Verification items for the finished model (mm, model axes). A direction names the side the tool comes from. Coordinates: 2 decimals unless noted, no trailing zeros. Order: outer loops, then holes, each group sorted by start corner. A loop starts at its lowest first (then second) coordinate and runs counter-clockwise, first axis right, second up. Notation, with made-up numbers: M -7.75,62.25 L 23.25,62.25 A17 ccw 23.25,88.25 Z; hole C 81.5,-22 d3. An arc over 180 degrees is marked long. Write item = value, one per line.
```python
from build123d import *
from OCP.BRepFilletAPI import BRepFilletAPI_MakeChamfer

# Parameters (mm, degrees)
SKETCH_1_W          = 200
SKETCH_1_H          = 230
EXTRUDE_1_DEPTH     = 20
CUT_EXTRUDE_1_REACH = 155.704
SKETCH_2_R          = 7
CHAMFER_1_SIZE      = 5
CHAMFER_1_SIZE2     = 3.501037691


with BuildPart() as part:
    # 草图1 → 凸台-拉伸1 (new body)
    with BuildSketch(Plane.XY):
        Rectangle(SKETCH_1_W, SKETCH_1_H)
    extrude(amount=EXTRUDE_1_DEPTH)

    # 草图2 → 切除-拉伸1 (cut, up to next)
    with BuildSketch(Plane.XY.offset(20), mode=Mode.PRIVATE) as cut_extrude_1_sk1:
        with Locations((-70, 95)):
            Circle(SKETCH_2_R)
    cut_extrude_1_tool1 = extrude(cut_extrude_1_sk1.sketch, amount=-CUT_EXTRUDE_1_REACH, mode=Mode.PRIVATE) & part.part
    # 草图2 → 切除-拉伸1 (cut, up to next)
    with BuildSketch(Plane.XY.offset(20), mode=Mode.PRIVATE) as cut_extrude_1_sk2:
        with Locations((0, 95)):
            Circle(SKETCH_2_R)
    cut_extrude_1_tool2 = extrude(cut_extrude_1_sk2.sketch, amount=-CUT_EXTRUDE_1_REACH, mode=Mode.PRIVATE) & part.part
    # 草图2 → 切除-拉伸1 (cut, up to next)
    with BuildSketch(Plane.XY.offset(20), mode=Mode.PRIVATE) as cut_extrude_1_sk3:
        with Locations((70, 95)):
            Circle(SKETCH_2_R)
    cut_extrude_1_tool3 = extrude(cut_extrude_1_sk3.sketch, amount=-CUT_EXTRUDE_1_REACH, mode=Mode.PRIVATE) & part.part
    # 草图2 → 切除-拉伸1 (cut, up to next)
    with BuildSketch(Plane.XY.offset(20), mode=Mode.PRIVATE) as cut_extrude_1_sk4:
        with Locations((-70, 35)):
            Circle(SKETCH_2_R)
    cut_extrude_1_tool4 = extrude(cut_extrude_1_sk4.sketch, amount=-CUT_EXTRUDE_1_REACH, mode=Mode.PRIVATE) & part.part
    # 草图2 → 切除-拉伸1 (cut, up to next)
    with BuildSketch(Plane.XY.offset(20), mode=Mode.PRIVATE) as cut_extrude_1_sk5:
        with Locations((70, 35)):
            Circle(SKETCH_2_R)
    cut_extrude_1_tool5 = extrude(cut_extrude_1_sk5.sketch, amount=-CUT_EXTRUDE_1_REACH, mode=Mode.PRIVATE) & part.part
    # 草图2 → 切除-拉伸1 (cut, up to next)
    with BuildSketch(Plane.XY.offset(20), mode=Mode.PRIVATE) as cut_extrude_1_sk6:
        with Locations((-70, -35)):
            Circle(SKETCH_2_R)
    cut_extrude_1_tool6 = extrude(cut_extrude_1_sk6.sketch, amount=-CUT_EXTRUDE_1_REACH, mode=Mode.PRIVATE) & part.part
    # 草图2 → 切除-拉伸1 (cut, up to next)
    with BuildSketch(Plane.XY.offset(20), mode=Mode.PRIVATE) as cut_extrude_1_sk7:
        with Locations((0, -95)):
            Circle(SKETCH_2_R)
    cut_extrude_1_tool7 = extrude(cut_extrude_1_sk7.sketch, amount=-CUT_EXTRUDE_1_REACH, mode=Mode.PRIVATE) & part.part
    # 草图2 → 切除-拉伸1 (cut, up to next)
    with BuildSketch(Plane.XY.offset(20), mode=Mode.PRIVATE) as cut_extrude_1_sk8:
        with Locations((-70, -95)):
            Circle(SKETCH_2_R)
    cut_extrude_1_tool8 = extrude(cut_extrude_1_sk8.sketch, amount=-CUT_EXTRUDE_1_REACH, mode=Mode.PRIVATE) & part.part
    # 草图2 → 切除-拉伸1 (cut, up to next)
    with BuildSketch(Plane.XY.offset(20), mode=Mode.PRIVATE) as cut_extrude_1_sk9:
        with Locations((70, -35)):
            Circle(SKETCH_2_R)
    cut_extrude_1_tool9 = extrude(cut_extrude_1_sk9.sketch, amount=-CUT_EXTRUDE_1_REACH, mode=Mode.PRIVATE) & part.part
    # 草图2 → 切除-拉伸1 (cut, up to next)
    with BuildSketch(Plane.XY.offset(20), mode=Mode.PRIVATE) as cut_extrude_1_sk10:
        with Locations((70, -95)):
            Circle(SKETCH_2_R)
    cut_extrude_1_tool10 = extrude(cut_extrude_1_sk10.sketch, amount=-CUT_EXTRUDE_1_REACH, mode=Mode.PRIVATE) & part.part
    # 草图2 → 切除-拉伸1 (cut, up to next)
    with BuildSketch(Plane.XY.offset(20), mode=Mode.PRIVATE) as cut_extrude_1_sk11:
        with BuildLine():
            Line((-41, 76), (41, 76))
            ThreePointArc((41, 76), (48.071067812, 73.071067812), (51, 66))
            Line((51, 66), (51, -66))
            ThreePointArc((51, -66), (48.071067812, -73.071067812), (41, -76))
            Line((41, -76), (-41, -76))
            ThreePointArc((-41, -76), (-48.071067812, -73.071067812), (-51, -66))
            Line((-51, -66), (-51, 66))
            ThreePointArc((-51, 66), (-48.071067812, 73.071067812), (-41, 76))
        make_face()
    cut_extrude_1_tool11 = extrude(cut_extrude_1_sk11.sketch, amount=-CUT_EXTRUDE_1_REACH, mode=Mode.PRIVATE) & part.part
    add(cut_extrude_1_tool1.solids().sort_by_distance((-70, 95, 20))[0], mode=Mode.SUBTRACT)
    add(cut_extrude_1_tool2.solids().sort_by_distance((0, 95, 20))[0], mode=Mode.SUBTRACT)
    add(cut_extrude_1_tool3.solids().sort_by_distance((70, 95, 20))[0], mode=Mode.SUBTRACT)
    add(cut_extrude_1_tool4.solids().sort_by_distance((-70, 35, 20))[0], mode=Mode.SUBTRACT)
    add(cut_extrude_1_tool5.solids().sort_by_distance((70, 35, 20))[0], mode=Mode.SUBTRACT)
    add(cut_extrude_1_tool6.solids().sort_by_distance((-70, -35, 20))[0], mode=Mode.SUBTRACT)
    add(cut_extrude_1_tool7.solids().sort_by_distance((0, -95, 20))[0], mode=Mode.SUBTRACT)
    add(cut_extrude_1_tool8.solids().sort_by_distance((-70, -95, 20))[0], mode=Mode.SUBTRACT)
    add(cut_extrude_1_tool9.solids().sort_by_distance((70, -35, 20))[0], mode=Mode.SUBTRACT)
    add(cut_extrude_1_tool10.solids().sort_by_distance((70, -95, 20))[0], mode=Mode.SUBTRACT)
    add(cut_extrude_1_tool11.solids().sort_by_distance((0, 0, 20))[0], mode=Mode.SUBTRACT)

    # 倒角1: one chamfer whose edges measure the first distance from different faces: ONE call of the kernel's chamfer builder (chamfer() names one face for all edges)
    chamfer_1_edges_1 = [part.edges().sort_by_distance(p)[0] for p in [
        (0, -115, 20),
    ]]
    chamfer_1_side_1 = [part.faces().sort_by_distance(p)[0] for p in [
        (0, -115, 10),
    ]]
    chamfer_1_edges_2 = [part.edges().sort_by_distance(p)[0] for p in [
        (0, 115, 20),
    ]]
    chamfer_1_side_2 = [part.faces().sort_by_distance(p)[0] for p in [
        (0, 115, 10),
    ]]
    chamfer_1 = BRepFilletAPI_MakeChamfer(part.part.solid().wrapped)
    for e in chamfer_1_edges_1:
        chamfer_1.Add(CHAMFER_1_SIZE, CHAMFER_1_SIZE2, e.wrapped, chamfer_1_side_1[0].wrapped)  # the first distance lies on this face
    for e in chamfer_1_edges_2:
        chamfer_1.Add(CHAMFER_1_SIZE, CHAMFER_1_SIZE2, e.wrapped, chamfer_1_side_2[0].wrapped)  # the first distance lies on this face
    add(Compound.cast(chamfer_1.Shape()), mode=Mode.REPLACE)


solid = part.part
```
Item 1: Release check for a two-part mould opening along X. For faces 3 (the flat face through (-1.4, 113.22, 17.54)), 4 (the flat face through (100, -2, 10)), 5 (the cylindrical face through (-0.91, 101.94, 10.14)) record: pulls with the +X half, pulls with the -X half, needs draft (parallel to the pull), parting line crosses it, or undercut.
Report:
face_3 = needs draft
face_4 = pulls with the +X half
face_5 = undercut
Item 2: Sectioned sample at A-A, the plane y = -35. Enter the section's corners in (x, z), then the cut area to 3 significant figures.
Report:
outline = M -100,0 L -77,0 L -77,20 L -100,20 Z; M -63,0 L -51,0 L -51,20 L -63,20 Z; M 51,0 L 63,0 L 63,20 L 51,20 Z; M 77,0 L 100,0 L 100,20 L 77,20 Z
area = 1,400 mm^2
Item 3: Tool access check on faces 1 (the flat face through (-1.4, -113.22, 17.54)), 2 (the cylindrical face through (-48.15, 72.99, 10.14)). Record the directions out of +Z, -Z, +X, -X, +Y, -Y that give a thin tool (end or side, any length) a straight path to the whole face; none if there is none.
Report:
face_1 = +Z, +X, -X, -Y
face_2 = +Z, -Z
Item 4: Scan lines: L1, parallel to Y at x = -70, z = 14.5; L2, parallel to Y at x = 0, z = 12.5; L3, parallel to Y at x = -32, z = 12.5. Record each from-to range of solid material in increasing order. Write a range as from..to.
Report:
L1 = -115..-102, -88..-42, -28..28, 42..88, 102..115
L2 = -115..-102, -88..-76, 76..88, 102..115
L3 = -115..-76, 76..115
Item 5: Sectioned sample at D-D, the plane x = 70. Enter the section's corners in (y, z).
Report:
outline = M -115,0 L -102,0 L -102,20 L -111.5,20 L -115,15 Z; M -88,0 L -42,0 L -42,20 L -88,20 Z; M -28,0 L 28,0 L 28,20 L -28,20 Z; M 42,0 L 88,0 L 88,20 L 42,20 Z; M 102,0 L 115,0 L 115,15 L 111.5,20 L 102,20 Z
Item 6: Gauge pin test, flat end, axial feed: pin 1 (8.5 mm diameter, centred on x = -70, y = 95, fed in from -Z). Record the tip position at first contact, or that the pin passes through.
Report:
pin_1 = through
Item 7: Sectioned sample at C-C, the plane y = 2. Enter the section's corners in (x, z), then the cut area to 3 significant figures.
Report:
outline = M -100,0 L -51,0 L -51,20 L -100,20 Z; M 51,0 L 100,0 L 100,20 L 51,20 Z
area = 1,960 mm^2
Item 8: Sectioned sample at B-B, the plane x = 0. Enter the section's corners in (y, z), then the cut area to 3 significant figures.
Report:
outline = M -115,0 L -102,0 L -102,20 L -111.5,20 L -115,15 Z; M -88,0 L -76,0 L -76,20 L -88,20 Z; M 76,0 L 88,0 L 88,20 L 76,20 Z; M 102,0 L 115,0 L 115,15 L 111.5,20 L 102,20 Z
area = 982 mm^2
